For this review, use the dimensioned drawing (mm, ordinates from the lowest corner) and the shaded views. A direction names the side the tool comes from. Give positions to 0.01 mm unless a question says otherwise; leave off trailing zeros. Write each loop counter-clockwise with the first axis right and the second up, starting at its lowest first coordinate (ties: lowest second). Pieces come first, ordered by that corner, then holes. Notation, with made-up numbers: (35, 17.5) -> (55, 17.5) arc R36 cw to (55, 54.5) -> close; hole circle Ø11 at (77, 89). An arc over 180 degrees is marked (long way). Return JSON: item names as keys, results as strings.
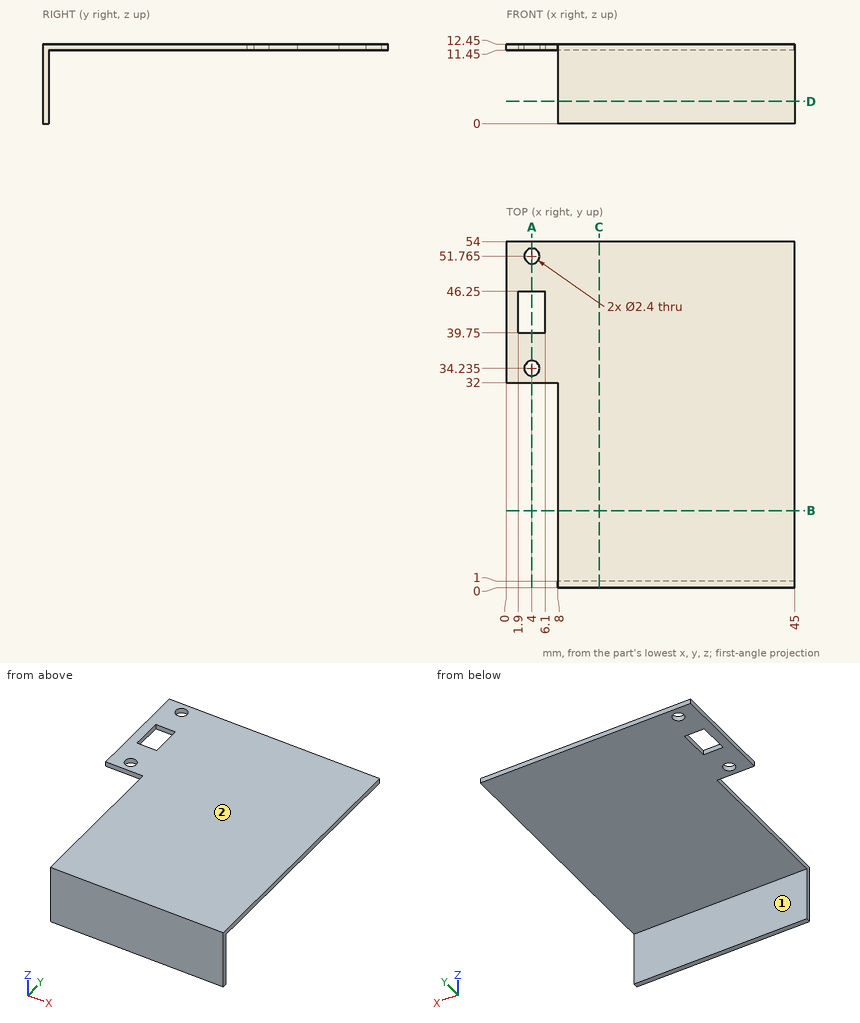
1. Add section C-C, the plane x = 14.5. State the section outline as (y, z) points.
Results found:
{"outline": "(0, 0) -> (1, 0) -> (1, 11.45) -> (54, 11.45) -> (54, 12.45) -> (0, 12.45) -> close"}
2. Add section D-D, the plane z = 3.5. State the section outline as (x, y) points.
Results found:
{"outline": "(8, 0) -> (45, 0) -> (45, 1) -> (8, 1) -> close"}
3. Add section A-A, the plane x = 4. State the section outline as (y, z) points (3 decimals).
Results found:
{"outline": "(32, 11.45) -> (33.035, 11.45) -> (33.035, 12.45) -> (32, 12.45) -> close; (35.435, 11.45) -> (39.75, 11.45) -> (39.75, 12.45) -> (35.435, 12.45) -> close; (46.25, 11.45) -> (50.565, 11.45) -> (50.565, 12.45) -> (46.25, 12.45) -> close; (52.965, 11.45) -> (54, 11.45) -> (54, 12.45) -> (52.965, 12.45) -> close"}
4. For pin 1 (0.5 mm diameter, centred on x = 3.5, z = 12, fed in from -Y), flat-tipped, find the tip position at first contact; note if it passes through.
Results found:
{"pin 1": "stops at y = 32"}
5. Add section B-B, the plane y = 12. State the section outline as (x, z) points, plus the area to 3 significant figures.
Results found:
{"outline": "(8, 11.45) -> (45, 11.45) -> (45, 12.45) -> (8, 12.45) -> close", "area": "37.0 mm²"}
6. To check wall thickness, follow probe 1 along Y at (x, z) = (4, 11.95) (3 decimals); probe 2 along Y at (x, z) = (38, 8); probe 3 along Z at (x, y) = (11.5, 24.5). State the ranges of each line that lie inside material, in increasing order.
Results found:
{"probe 1": "y = 32 to 33.035, 35.435 to 39.75, 46.25 to 50.565, 52.965 to 54", "probe 2": "y = 0 to 1", "probe 3": "z = 11.45 to 12.45"}
7. For the marked faces 1 and 2, list the 3-axis set-ups (+Z, -Z, +X, -X, +Y, -Y) from which the entire face can be reached by the end or side of a thin tool; tool diameter is ignored.
Results found:
{"face 1": "-Z, +X, -X, +Y", "face 2": "+Z, +X, -X, +Y, -Y"}
